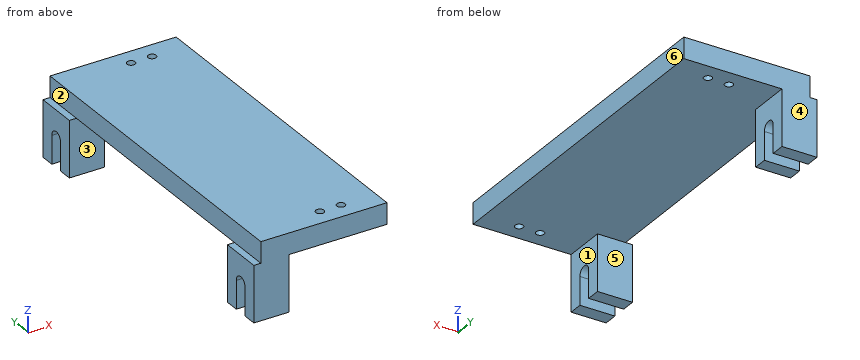
from build123d import *

# Parameters (mm, degrees)
SKETCH011_W              = 240
SKETCH011_H              = 15
PAD007_DEPTH             = 90
SKETCH012_R              = 2.9
HOLE004_DEPTH            = 270.001
PAD008_DEPTH             = 25
CLONE007_PLACEMENT_ANGLE = 180


with BuildPart() as part:
    # Sketch011 → Pad007 (new body)
    with BuildSketch(Plane.YZ.offset(5)):
        with Locations((95, 262.5)):
            Rectangle(SKETCH011_W, SKETCH011_H)
    extrude(amount=PAD007_DEPTH)

    # Sketch012 → Hole004 (cut, through all)
    with BuildSketch(Plane.XY):
        with Locations((55, 202.5)):
            Circle(SKETCH012_R)
        with Locations((70, 202.5)):
            Circle(SKETCH012_R)
        with Locations((55, -12.5)):
            Circle(SKETCH012_R)
        with Locations((70, -12.5)):
            Circle(SKETCH012_R)
    extrude(amount=HOLE004_DEPTH, mode=Mode.SUBTRACT)

    # Sketch013 → Pad008 (join)
    with BuildSketch(Plane.YZ):
        with BuildLine():
            Line((-25, 270), (-25, 310))
            Line((-15, 310), (-25, 310))
            Line((-15, 310), (-15, 290))
            ThreePointArc((-15, 290), (-10, 285), (-5, 290))
            Line((-5, 310), (-5, 290))
            Line((-5, 310), (5, 310))
            Line((5, 270), (5, 310))
            Line((-25, 270), (5, 270))
        make_face()
        with BuildLine():
            Line((185, 270), (185, 310))
            Line((195, 310), (185, 310))
            Line((195, 310), (195, 290))
            ThreePointArc((195, 290), (200, 285), (205, 290))
            Line((205, 310), (205, 290))
            Line((205, 310), (215, 310))
            Line((215, 270), (215, 310))
            Line((185, 270), (215, 270))
        make_face()
    extrude(amount=PAD008_DEPTH)


with BuildPart() as part_1:
    # Clone007 placement: moved
    add(part.part.moved(Location((0, 190, 260))).rotate(Axis((0, 190, 260), (1, 0, 0)), CLONE007_PLACEMENT_ANGLE))


solid = part_1.part
The listing builds one solid part. Answer for the finished solid, in the listing's coordinates (mm). Face numbers are marked on the shaded views. A direction names the side the tool comes from. Round coordinates to 2 decimals unless told otherwise and drop trailing zeros. Write each loop counter-clockwise with the first axis right and the second up, starting at its lowest first coordinate (ties: lowest second). Pieces come first, ordered by that corner, then holes. Notation, with made-up numbers: (-23, 12.5) - (26, 12.5) arc R18 ccw to (26, 31.5) - close; hole circle Ø4 at (59.25, 34.5). An arc over 180 degrees is marked (long way). Use a Markdown table: item, result. Add a question column.
1. For a pull along Y with two mould halves and no side action, classify the marked faces 4, 5 and 6 as +Y half, -Y half, draft (parallel to the pull), parting line (faces both ways), or undercut.
2. Consider line 1 (X direction, y = 202, z = -1); line 2 (Y direction, x = 70, z = 1.75); line 3 (Z direction, x = 90.5, y = 137). Determine where each line is inside the solid, lowest interval first.
3. The part is cut by section D-D (y = -12.5). Write down the section's boundary in (x, z).
4. The part is cut by section B-B (x = 70). Write down the section's boundary in (y, z).
5. A tool of negligible diameter and unlimited length cuts with its end or side. For the marked faces 1, 2 and 3, from which of +Z, -Z, +X, -X, +Y, -Y can it reach the whole face along a straight path? Write none if from no direction.
6. Flat-ended cylindrical pins translate along their axes: P1, Ø1.5, axis at x = 1.5, y = 201, coming from the +Z side; P2, Ø5, axis at x = 60, y = 151, coming from the -Z side; P3, Ø4.5, axis at y = 85, z = 0, coming from the -X side. Find the tip coordinate at first contact, or state that the pin passes through.
7. The part is cut by section A-A (z = -18.5). Write down the section's boundary in (x, y), and give its area (3 significant figures).
8. The part is cut by section C-C (z = -42). Write down the section's boundary in (x, y).
Reported:
| question | item | result |
|---|---|---|
| 1 | face 4 | +Y half |
| 1 | face 5 | undercut |
| 1 | face 6 | draft |
| 2 | line 1 | 5 to 52.14, 57.86 to 67.14, 72.86 to 95 |
| 2 | line 2 | -25 to -15.4, -9.6 to 199.6, 205.4 to 215 |
| 2 | line 3 | -10 to 5 |
| 3 | outline | (0, -25.67) - (25, -25.67) - (25, -10) - (52.1, -10) - (52.1, 5) - (5, 5) - (5, -10) - (0, -10) - close; (57.9, -10) - (67.1, -10) - (67.1, 5) - (57.9, 5) - close; (72.9, -10) - (95, -10) - (95, 5) - (72.9, 5) - close |
| 4 | outline | (-25, -10) - (-15.4, -10) - (-15.4, 5) - (-25, 5) - close; (-9.6, -10) - (199.6, -10) - (199.6, 5) - (-9.6, 5) - close; (205.4, -10) - (215, -10) - (215, 5) - (205.4, 5) - close |
| 5 | face 1 | -Z, +X, +Y, -Y |
| 5 | face 2 | +Z, -X, +Y, -Y |
| 5 | face 3 | -Z, +X, -X |
| 6 | P1 | z = -10 |
| 6 | P2 | z = -10 |
| 6 | P3 | x = 5 |
| 7 | outline | (0, -25) - (25, -25) - (25, 5) - (0, 5) - close; (0, 185) - (25, 185) - (25, 215) - (0, 215) - close |
| 7 | area | 1,500 mm^2 |
| 8 | outline | (0, -25) - (25, -25) - (25, -15) - (0, -15) - close; (0, -5) - (25, -5) - (25, 5) - (0, 5) - close; (0, 185) - (25, 185) - (25, 195) - (0, 195) - close; (0, 205) - (25, 205) - (25, 215) - (0, 215) - close |
